Can you work these out from the model? Positions are in its coordinate system, mm. Face numbers are marked on the shaded views. A direction names the side the tool comes from. Give positions to 0.01 mm unless a question says otherwise; leave off trailing zeros. Write each loop counter-clockwise with the first axis right and the second up, starting at its lowest first coordinate (ties: lowest second). Pieces come first, ordered by that corner, then holes.
```python
from build123d import *

# Parameters (mm, degrees)
F1_DEPTH = 25.4


with BuildPart() as f1:
    # F0 (on Front) → F1 (new body)
    with BuildSketch(Plane.XZ):
        Polygon((36.621895, 34.384649), (0, 55.268008), (-38.276557, 34.384649), (-29.714473, 34.384649), (-17.944092, 34.384649), align=None)
        Polygon((-38.276557, 26.495456), (-38.276557, 34.384649), (-52.73645, 26.495456), align=None)
        Polygon((-29.714473, 34.384649), (-38.276557, 34.384649), (-38.276557, 26.495456), (-38.276557, 0), (-29.714473, 0), (-16.381497, 0), (12.651484, 0), (36.621895, 0), (36.621895, 27.243869), (36.621895, 33.672655), (36.621895, 34.384649), (-17.944092, 34.384649), align=None)
        Polygon((47.895672, 27.243869), (36.621895, 34.384649), (36.621895, 33.672655), align=None)
        Polygon((47.895672, 27.243869), (36.621895, 33.672655), (36.621895, 27.243869), align=None)
        Polygon((12.651484, 0), (-16.381497, 0), (-16.381497, -57.907131), (-16.381497, -63.601866), (14.517904, -63.601866), (12.651484, -60.177624), align=None)
    extrude(amount=F1_DEPTH)


solid = f1.part
```
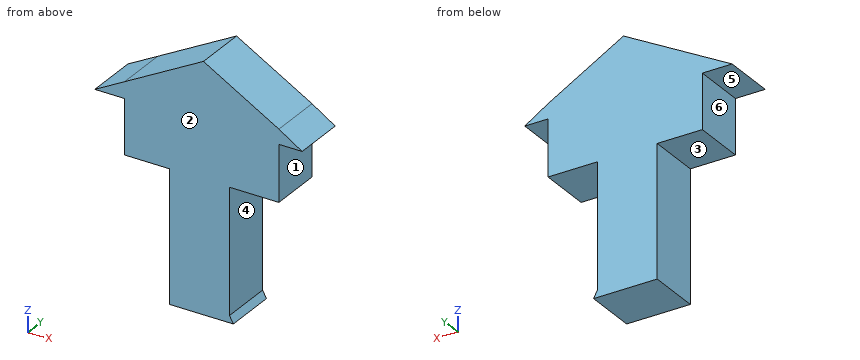
1) Suppose I cut it at A-A on y = -11. Write out the boundary of the cut face in (x, z), plus the area to 3 significant figures.
Values follow:
outline: (-52.74, 26.5) - (-38.28, 26.5) - (-38.28, 0) - (-16.38, 0) - (-16.38, -63.6) - (14.52, -63.6) - (12.65, -60.18) - (12.65, 0) - (36.62, 0) - (36.62, 27.24) - (47.9, 27.24) - (36.62, 34.38) - (0, 55.27) - close
area: 5,300 mm2
2) For the marked faces 1, 2 and 3, which set-ups out of +Z, -Z, +X, -X, +Y, -Y let a thin tool reach every point of the face, with its end or its side?
Values follow:
face 1: -Z, +X, +Y, -Y
face 2: +Z, -Z, +X, -X, -Y
face 3: -Z, -X, +Y, -Y
3) Suppose I cut it at C-C on x = 22. Write out the boundary of the cut face in (y, z).
Values follow:
outline: (-25.4, 0) - (0, 0) - (0, 42.72) - (-25.4, 42.72) - close
4) Suppose I cut it at B-B on z = -47. Write out the boundary of the cut face in (x, y), plus the area to 3 significant figures.
Values follow:
outline: (-16.38, -25.4) - (12.65, -25.4) - (12.65, 0) - (-16.38, 0) - close
area: 737 mm2
5) For pin 1 Ø8 at (x, y) = (-6, -12.5) entering from +Z; pin 2 Ø7.5 at (y, z) = (-18, -37) entering from +X; pin 3 Ø6 at (x, y) = (21.5, -3.5) entering from +Z, each with a flat end and sliding along its axis, tell me the tip position at first contact or that it passes through.
Values follow:
pin 1: stops at z = 54.18
pin 2: stops at x = 12.65
pin 3: stops at z = 44.72
6) Please list where these lines run through material, in increasing order: L1, parallel to X at y = -22.5, z = -5.5; L2, parallel to X at y = -8, z = 1.5; L3, parallel to Z at x = -20.5, y = -5.5.
Values follow:
L1: x = -16.38 to 12.65
L2: x = -38.28 to 36.62
L3: z = 0 to 44.08
7) If we mould it in two halves opening along Z, with no side actions, what happens to the marked faces 4, 5 and 6? For each: +Z half, -Z half, draft (parallel to the pull), parting line (faces both ways), or undercut.
Values follow:
face 4: undercut
face 5: -Z half
face 6: draft
